For this review, use the dimensioned drawing (mm, ordinates from the lowest corner) and the shaded views. Give positions to 0.01 mm unless a question says otherwise; leave off trailing zeros. Order: outer loops, then holes, each group sorted by start corner. A loop starts at its lowest first (then second) coordinate and runs counter-clockwise, first axis right, second up. Notation, with made-up numbers: (2.5, -31.5) - (54.5, -31.5) arc R27 ccw to (54.5, 6.5) - close; hole circle Ø5 at (55, 13). An arc over 180 degrees is marked (long way). One line per item, written item: value.
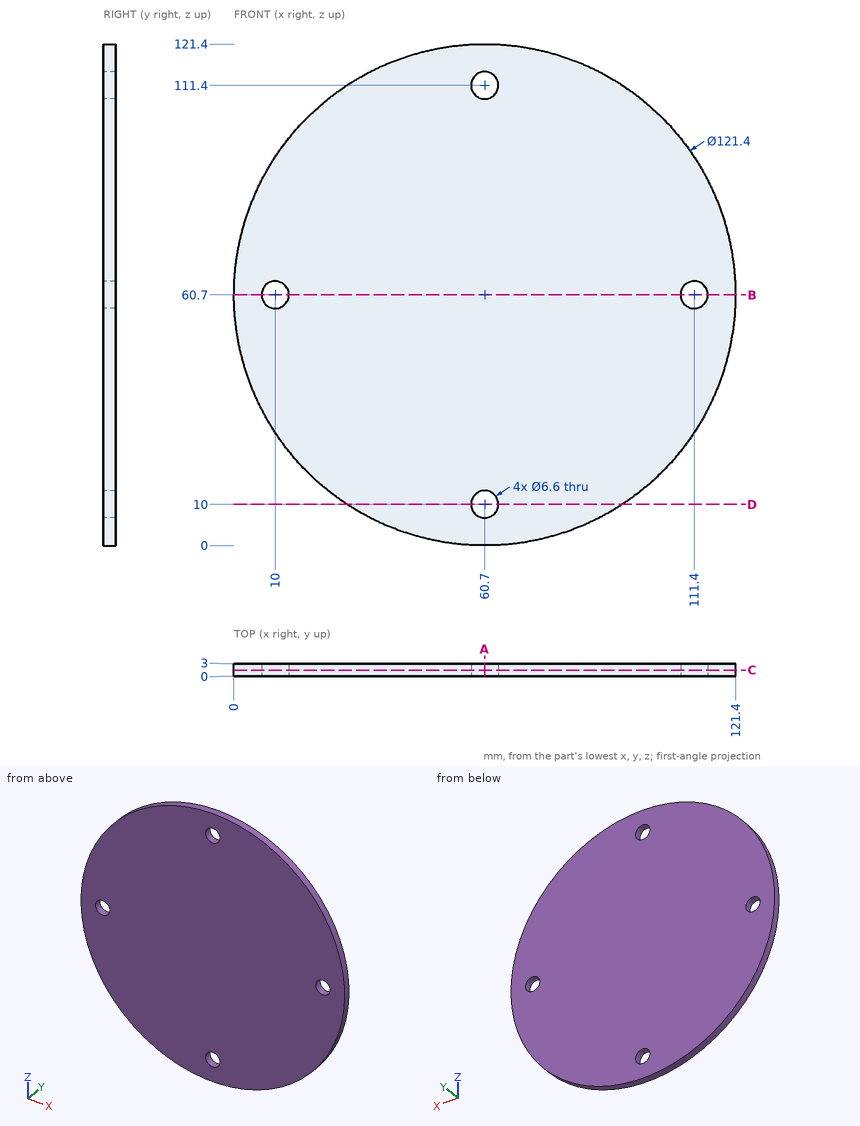
(1) Take a section at D-D (z = 10). Write out the cut boundary in (x, y).
Answers below:
outline: (27.32, 0) - (57.4, 0) - (57.4, 3) - (27.32, 3) - close; (64, 0) - (94.08, 0) - (94.08, 3) - (64, 3) - close
(2) Take a section at A-A (x = 60.7). Write out the cut boundary in (y, z).
Answers below:
outline: (0, 0) - (3, 0) - (3, 6.7) - (0, 6.7) - close; (0, 13.3) - (3, 13.3) - (3, 108.1) - (0, 108.1) - close; (0, 114.7) - (3, 114.7) - (3, 121.4) - (0, 121.4) - close
(3) Wall thickness on line 1 (X direction, y = 1.65, z = 113); line 2 (Z direction, x = 54, y = 2.7); line 3 (Z direction, x = 108.5, y = 1.7): over which ranges is each line inside the solid? List them lowest first. Write a range as from..to.
Answers below:
line 1: x = 29.89..57.81, 63.59..91.51
line 2: z = 0.37..121.03
line 3: z = 23.29..59.13, 62.27..98.11
(4) Take a section at B-B (z = 60.7). Write out the cut boundary in (x, y), then the cut area to 3 significant figures.
Answers below:
outline: (0, 0) - (6.7, 0) - (6.7, 3) - (0, 3) - close; (13.3, 0) - (108.1, 0) - (108.1, 3) - (13.3, 3) - close; (114.7, 0) - (121.4, 0) - (121.4, 3) - (114.7, 3) - close
area: 325 mm^2
(5) Take a section at C-C (y = 1.4). Write out the cut boundary in (x, z).
Answers below:
outline: circle Ø121.4 at (60.7, 60.7); hole circle Ø6.6 at (10, 60.7); hole circle Ø6.6 at (60.7, 10); hole circle Ø6.6 at (60.7, 111.4); hole circle Ø6.6 at (111.4, 60.7)
